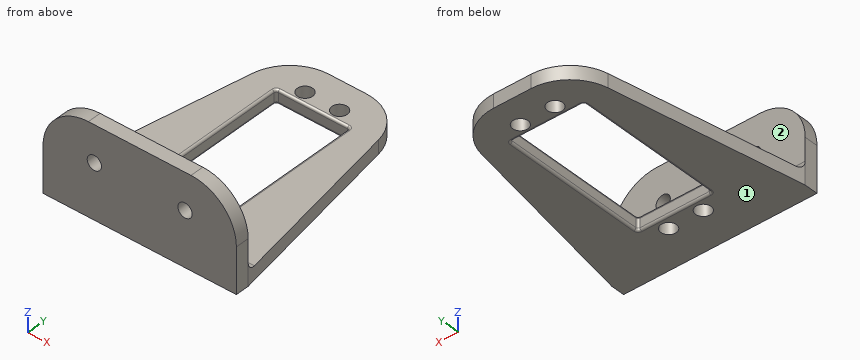
```python
from build123d import *

# Parameters (mm, degrees)
FILLET2_START       = -0.929916211
FILLET2_OUTLINE_R   = 2.15
FILLET2_DEPTH       = 3.81
FILLET2_START_2     = 2.880083789
FILLET2_2_OUTLINE_W = 54.14352655
FILLET2_2_OUTLINE_H = 3.81
FILLET2_2_DEPTH     = 34.29
FILLET6_R           = 2.54
SKETCH6_W           = 54.14352655
SKETCH6_H           = 3.81
CUT_EXTRUDE2_DEPTH  = 12.7
FILLET8_R           = 12.7
SKETCH7_R           = 1.999996
CUT_EXTRUDE3_DEPTH  = 76.817206459
SKETCH8_W           = 20.6375
SKETCH8_H           = 41.275
CUT_EXTRUDE5_DEPTH  = 69.202637613
FILLET10_R          = 0.635


with BuildPart() as part:
    # Fillet2: read off the stored shape, not the designer's step
    # Fillet2 outline → Fillet2 (new body)
    with BuildSketch(Plane.XY.offset(FILLET2_START)):
        with BuildLine():
            Line((20.718778313, -51.581857548), (11.372508186, 1.423474309))
            ThreePointArc((11.372508186, 1.423474309), (7.028852365, 8.94690688), (-1.134550278, 11.918142452))
            Line((-1.134550278, 11.918142452), (-11.571419646, 11.918142452))
            ThreePointArc((-11.571419646, 11.918142452), (-19.734822289, 8.94690688), (-24.078478109, 1.423474309))
            Line((-24.078478109, 1.423474309), (-33.424748237, -51.581857548))
            Line((-33.424748237, -51.581857548), (-33.424748237, -55.391857548))
            Line((-33.424748237, -55.391857548), (20.718778313, -55.391857548))
            Line((20.718778313, -55.391857548), (20.718778313, -51.581857548))
        make_face()
        with Locations((-11.306344138, -44.161858203)):
            Circle(FILLET2_OUTLINE_R, mode=Mode.SUBTRACT)
        with Locations((-1.606344138, -44.161858203)):
            Circle(FILLET2_OUTLINE_R, mode=Mode.SUBTRACT)
        with Locations((-11.306344138, 3.838143108)):
            Circle(FILLET2_OUTLINE_R, mode=Mode.SUBTRACT)
        with Locations((-1.606344138, 3.838143108)):
            Circle(FILLET2_OUTLINE_R, mode=Mode.SUBTRACT)
    extrude(amount=FILLET2_DEPTH)

    # Fillet2 2 outline → Fillet2 2 (add)
    with BuildSketch(Plane.XY.offset(FILLET2_START_2)):
        with Locations((-6.352984962, -53.486857548)):
            Rectangle(FILLET2_2_OUTLINE_W, FILLET2_2_OUTLINE_H)
    extrude(amount=FILLET2_2_DEPTH)

    # Fillet6
    fillet6_edges = [part.edges().sort_by_distance(p)[0] for p in [
        (-6.352984962, -51.581857548, 2.880083789),
    ]]
    fillet(fillet6_edges, radius=FILLET6_R)

    # Sketch6 → Cut-Extrude2 (cut)
    with BuildSketch(Plane.XY.offset(37.170083789)):
        with Locations((-6.352984962, -53.486857548)):
            Rectangle(SKETCH6_W, SKETCH6_H)
    extrude(amount=-CUT_EXTRUDE2_DEPTH, mode=Mode.SUBTRACT)

    # Fillet8
    fillet8_edges = [part.edges().sort_by_distance(p)[0] for p in [
        (-33.424748237, -53.486857548, 24.470083789),
        (20.718778313, -53.486857548, 24.470083789),
    ]]
    fillet(fillet8_edges, radius=FILLET8_R)

    # Sketch7 → Cut-Extrude3 (cut, through all)
    with BuildSketch(Plane(origin=(0, -51.581857548, 0), x_dir=(1, 0, 0), z_dir=(0, 1, 0))):
        with Locations(Location((-19.052984962, -14.310083789, 0), (0, 0, 270))):
            Circle(SKETCH7_R)
        with Locations(Location((6.347015038, -14.310083789, 0), (0, 0, 90))):
            Circle(SKETCH7_R)
    extrude(amount=-CUT_EXTRUDE3_DEPTH, mode=Mode.SUBTRACT)

    # Sketch8 → Cut-Extrude5 (cut, through all)
    with BuildSketch(Plane.XY.offset(2.880083789)):
        with Locations((-6.352984962, -19.974356892)):
            Rectangle(SKETCH8_W, SKETCH8_H)
    extrude(amount=-CUT_EXTRUDE5_DEPTH, mode=Mode.SUBTRACT)

    # Fillet10
    fillet10_edges = [part.edges().sort_by_distance(p)[0] for p in [
        (3.965765038, -19.974356892, 2.880083789),
        (3.965765038, 0.663143108, 0.975083789),
        (-6.352984962, -40.611856892, -0.929916211),
        (3.965765038, -40.611856892, 0.975083789),
        (-16.671734962, -19.974356892, -0.929916211),
        (-16.671734962, -40.611856892, 0.975083789),
        (-6.352984962, 0.663143108, 2.880083789),
        (-16.671734962, 0.663143108, 0.975083789),
        (3.965765038, -19.974356892, -0.929916211),
        (-6.352984962, 0.663143108, -0.929916211),
        (-16.671734962, -19.974356892, 2.880083789),
        (-6.352984962, -40.611856892, 2.880083789),
    ]]
    fillet(fillet10_edges, radius=FILLET10_R)


solid = part.part
```
Check sheet for the modelled part. Datum: model origin and axes. Units: mm. Face numbers are marked on the shaded views. A direction names the side the tool comes from. Coordinates: 2 decimals unless noted, no trailing zeros. Write each loop counter-clockwise with the first axis right and the second up, starting at its lowest first coordinate (ties: lowest second). Pieces come first, ordered by that corner, then holes. Notation, with made-up numbers: (59.5, -18.75) -> (106.5, -18.75) arc R18 cw to (106.5, -1.75) -> close; hole circle Ø6 at (85, -3.75). An arc over 180 degrees is marked (long way). Use a Markdown table: item, result.
1. Sectioned sample at A-A (x = -5.5). Enter the section's corners in (y, z) (3 decimals).
Reported:
| item | result |
|---|---|
| outline | (-55.392, -0.93) -> (-41.247, -0.93) arc R0.635 ccw to (-40.612, -0.295) -> (-40.612, 2.245) arc R0.635 ccw to (-41.247, 2.88) -> (-49.042, 2.88) arc R2.54 cw to (-51.582, 5.42) -> (-51.582, 24.47) -> (-55.392, 24.47) -> close; (0.663, -0.295) arc R0.635 ccw to (1.298, -0.93) -> (11.918, -0.93) -> (11.918, 2.88) -> (1.298, 2.88) arc R0.635 ccw to (0.663, 2.245) -> close |
2. Sectioned sample at B-B (y = -34.5). Enter the section's corners in (x, z) (3 decimals), plus the area to 3 significant figures.
Reported:
| item | result |
|---|---|
| outline | (-30.413, -0.93) -> (-17.307, -0.93) arc R0.635 ccw to (-16.672, -0.295) -> (-16.672, 2.245) arc R0.635 ccw to (-17.307, 2.88) -> (-30.413, 2.88) -> close; (3.966, -0.295) arc R0.635 ccw to (4.601, -0.93) -> (17.707, -0.93) -> (17.707, 2.88) -> (4.601, 2.88) arc R0.635 ccw to (3.966, 2.245) -> close |
| area | 104 mm2 |
3. Tool access check on the marked faces 1 and 2. Record the directions out of +Z, -Z, +X, -X, +Y, -Y that give a thin tool (end or side, any length) a straight path to the whole face; none if there is none.
Reported:
| item | result |
|---|---|
| face 1 | -Z, +X, -X, +Y, -Y |
| face 2 | +Z, +X, -X, +Y |
4. Scan lines: line 1 along Y through (x, z) = (-4, 7.5); line 2 along X through (y, z) = (-46, 0.5); line 3 along Z through (x, y) = (8, -15.5). Record each from-to range of solid material in increasing order.
Reported:
| item | result |
|---|---|
| line 1 | y = -55.39 to -51.58 |
| line 2 | x = -32.44 to -12.42, -10.19 to -2.72, -0.49 to 19.73 |
| line 3 | z = -0.93 to 2.88 |
5. Sectioned sample at C-C (x = 15). Enter the section's corners in (y, z), plus the area to 3 significant figures.
Reported:
| item | result |
|---|---|
| outline | (-55.39, -0.93) -> (-19.15, -0.93) -> (-19.15, 2.88) -> (-49.04, 2.88) arc R2.54 cw to (-51.58, 5.42) -> (-51.58, 22.38) -> (-55.39, 22.38) -> close |
| area | 214 mm2 |
6. Sectioned sample at D-D (z = 6.5). Enter the section's corners in (x, y).
Reported:
| item | result |
|---|---|
| outline | (-33.42, -55.39) -> (20.72, -55.39) -> (20.72, -51.58) -> (-33.42, -51.58) -> close |
7. Go/stop test with flat-tipped pins: pin 1 Ø5.5 at (x, y) = (-11.31, 3.84) entering from +Z; pin 2 Ø1.3 at (y, z) = (-22.5, 1.5) entering from +X; pin 3 Ø5.5 at (x, z) = (-3, 10.5) entering from +Y; pin 4 Ø6.5 at (x, z) = (-19.05, 14.31) entering from -Y. Record where each tip stops, or that it passes through.
Reported:
| item | result |
|---|---|
| pin 1 | stops at z = 2.88 |
| pin 2 | stops at x = 15.71 |
| pin 3 | stops at y = -51.58 |
| pin 4 | stops at y = -55.39 |
